Input: part model. Units: mm. Frame: model coordinates. Face numbers are marked on the shaded views. A direction names the side the tool comes from. Round coordinates to 2 decimals unless told otherwise and drop trailing zeros. Loops run counter-clockwise (first coordinate to the right, second up) from the corner with the lowest first, then second, coordinate; pieces in that order, holes last. Notation, with made-up numbers: (10, 61) -> (38, 61) arc R9 ccw to (38, 65) -> close; hole circle Ø11 at (14, -32). An arc over 180 degrees is marked (long way). Answer as a JSON object with one key per item and string values. Group by question number.
Item 1: Pin query (flat end, axial travel): pin 1 (8 mm diameter, centred on y = -2, z = -4, fed in from -X); pin 2 (4 mm diameter, centred on x = 8, z = 0, fed in from +Y); pin 3 (6 mm diameter, centred on y = 17, z = -4, fed in from +X). Return the tip coordinate at first contact, or that it passes through.
Item 2: Material intervals for line 1 (X direction, y = -4, z = 0); line 2 (Y direction, x = 1.5, z = -8.5); line 3 (Y direction, x = 2.5, z = -10.75), sorted ascending. Write a range as [from, to].
Item 3: Draft query along Y for the marked faces 3, 4, 5 and 6. Return one class per face: released by +Y, released by -Y, zero draft, split by the parting line, or undercut.
Item 4: Set-up query: the marked faces 1 and 2. Return all of +Z, -Z, +X, -X, +Y, -Y with unobstructed straight access to the full face (end or side cutting, diameter ignored); none if empty.
Item 5: Section query C-C on x = 3.75. Return loops of the section in (y, z).
Item 6: Section query A-A on z = 0. Return loops of the section in (x, y), and give its area (3 significant figures).
Item 7: Section query D-D on y = -1. Return loops of the section in (x, z).
Item 8: Section query B-B on x = 0. Return loops of the section in (y, z).
from build123d import *

# Parameters (mm, degrees)
SKETCH1_R           = 13.45
BOSS_EXTRUDE1_DEPTH = 13.9
SKETCH2_R           = 10
SKETCH2_R_2         = 1.5
BOSS_EXTRUDE3_DEPTH = 2.5
BOSS_EXTRUDE4_REACH = 27.578
SKETCH3_R           = 5
SKETCH4_R           = 2.5
BOSS_EXTRUDE5_DEPTH = 13.5


with BuildPart() as part:
    # Sketch1 → Boss-Extrude1 (new body)
    with BuildSketch(Plane(origin=(0, 0, 0), x_dir=(1, 0, 0), z_dir=(0, 1, 0))):
        with Locations(Location((0, 0, 0), (0, 0, 270))):
            Circle(SKETCH1_R)
    extrude(amount=BOSS_EXTRUDE1_DEPTH)

    # Sketch3 → Boss-Extrude4 (add, up to next)
    with BuildSketch(Plane(origin=(0, -3.2, 0), x_dir=(1, 0, 0), z_dir=(0, 1, 0)), mode=Mode.PRIVATE) as boss_extrude4_sk1:
        with Locations(Location((0, 0, 0), (0, 0, 270))):
            Circle(SKETCH3_R)
    boss_extrude4_tool1 = extrude(boss_extrude4_sk1.sketch, amount=BOSS_EXTRUDE4_REACH, mode=Mode.PRIVATE) - part.part


with BuildPart() as body_2:
    # Sketch2 → Boss-Extrude3 (new body)
    with BuildSketch(Plane.XZ.offset(5.7)):
        with Locations(Location((0, 0, 0), (0, 0, 270))):
            Circle(SKETCH2_R)
        with Locations(Location((0, 8, 0), (0, 0, 270))):
            Circle(SKETCH2_R_2, mode=Mode.SUBTRACT)
        with Locations(Location((8, 0, 0), (0, 0, 270))):
            Circle(SKETCH2_R_2, mode=Mode.SUBTRACT)
        with Locations(Location((0, -8, 0), (0, 0, 270))):
            Circle(SKETCH2_R_2, mode=Mode.SUBTRACT)
        with Locations(Location((-8, 0, 0), (0, 0, 270))):
            Circle(SKETCH2_R_2, mode=Mode.SUBTRACT)
    extrude(amount=-BOSS_EXTRUDE3_DEPTH)


with BuildPart() as part_1:
    add(part.part)

    add(body_2.part)  # Boss-Extrude4 merges body 2
    add(boss_extrude4_tool1.solids().sort_by_distance((0, -3.2, 0))[0])

    # Sketch4 → Boss-Extrude5 (add)
    with BuildSketch(Plane(origin=(0, 13.9, 0), x_dir=(1, 0, 0), z_dir=(0, 1, 0))):
        with Locations(Location((0, 0, 0), (0, 0, 270))):
            Circle(SKETCH4_R)
    extrude(amount=BOSS_EXTRUDE5_DEPTH)


solid = part_1.part
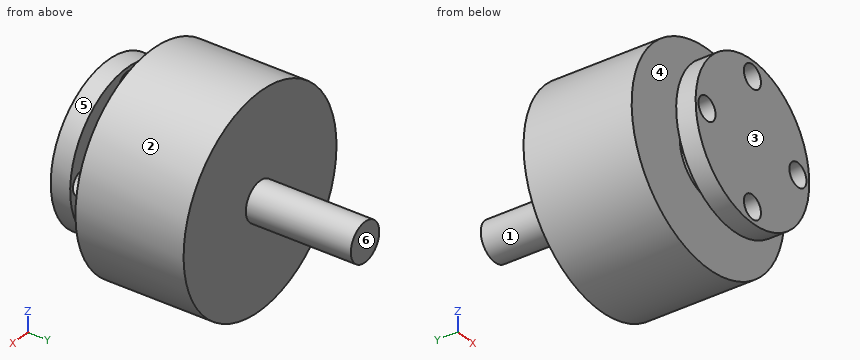
Solved:
{
 "1": {"pin 1": "x = -13.44", "pin 2": "y = 13.9", "pin 3": "x = 2.29"},
 "2": {"line 1": "[-10, -9.5], [-6.5, 6.5], [9.5, 10]", "line 2": "[-5.7, -3.2], [0, 13.9]", "line 3": "[0, 13.9]"},
 "3": {"face 3": "released by -Y", "face 4": "undercut", "face 5": "zero draft", "face 6": "released by +Y"},
 "4": {"face 1": "+Y", "face 2": "+Y, -Y"},
 "5": {"outline": "(-5.7, -9.27) -> (-3.2, -9.27) -> (-3.2, -3.31) -> (0, -3.31) -> (0, -12.92) -> (13.9, -12.92) -> (13.9, 12.92) -> (0, 12.92) -> (0, 3.31) -> (-3.2, 3.31) -> (-3.2, 9.27) -> (-5.7, 9.27) -> close"},
 "6": {"outline": "(-13.45, 0) -> (-5, 0) -> (-5, -3.2) -> (-6.5, -3.2) -> (-6.5, -5.7) -> (6.5, -5.7) -> (6.5, -3.2) -> (5, -3.2) -> (5, 0) -> (13.45, 0) -> (13.45, 13.9) -> (2.5, 13.9) -> (2.5, 27.4) -> (-2.5, 27.4) -> (-2.5, 13.9) -> (-13.45, 13.9) -> close; (-10, -5.7) -> (-9.5, -5.7) -> (-9.5, -3.2) -> (-10, -3.2) -> close; (9.5, -5.7) -> (10, -5.7) -> (10, -3.2) -> (9.5, -3.2) -> close", "area": "508 mm²"},
 "7": {"outline": "circle Ø10 at (0, 0)"},
 "8": {"outline": "(-5.7, -10) -> (-3.2, -10) -> (-3.2, -9.5) -> (-5.7, -9.5) -> close; (-5.7, -6.5) -> (-3.2, -6.5) -> (-3.2, -5) -> (0, -5) -> (0, -13.45) -> (13.9, -13.45) -> (13.9, -2.5) -> (27.4, -2.5) -> (27.4, 2.5) -> (13.9, 2.5) -> (13.9, 13.45) -> (0, 13.45) -> (0, 5) -> (-3.2, 5) -> (-3.2, 6.5) -> (-5.7, 6.5) -> close; (-5.7, 9.5) -> (-3.2, 9.5) -> (-3.2, 10) -> (-5.7, 10) -> close"}
}
